```python
from build123d import *

# Parameters (mm, degrees)
F0_R          = 1.5
F0_R_2        = 4.5
F1_DEPTH      = 3
F2_W          = 12
F2_H          = 29
F3_DEPTH      = 3
F4_R          = 1.5
F5_DEPTH      = 3
F6_R          = 4
F6_R_2        = 1.5
F7_DEPTH      = 3
F9_R          = 2
F10_T4_DEPTH  = 12
F10_S5_R      = 1.5
F10_T6_DEPTH  = 8
F10_T10_DEPTH = 12
F10_S11_R     = 1.5
F10_T12_DEPTH = 8
F11_R         = 3
F12_DEPTH     = 4
F13_R         = 0.5
F14_DEPTH     = 3
F15_T1_DEPTH  = 8
F16_T1_DEPTH  = 8
F17_SIZE      = 2


# Not quite as in the source:
# - a fillet or chamfer that OpenCascade refuses, or shapes differently, is made with other operations: its cross-section is extruded or revolved along the edge and cut away or added


with BuildPart() as f1:
    # F0 (on Front) → F1 (new body)
    with BuildSketch(Plane.XZ):
        with BuildLine():
            Line((0, -5.5), (9.5, -5.5))
            ThreePointArc((9.5, -5.5), (11.6605151609, -5.0578823869), (13.4736842105, -3.8026088144))
            ThreePointArc((13.4736842105, -3.8026088144), (14, 0), (13.4736842105, 3.8026088144))
            ThreePointArc((13.4736842105, 3.8026088144), (11.6605151609, 5.0578823869), (9.5, 5.5))
            Line((9.5, 5.5), (0, 5.5))
            Line((0, 5.5), (-9.5, 5.5))
            ThreePointArc((-9.5, 5.5), (-11.6605151609, 5.0578823869), (-13.4736842105, 3.8026088144))
            ThreePointArc((-13.4736842105, 3.8026088144), (-14, 0), (-13.4736842105, -3.8026088144))
            ThreePointArc((-13.4736842105, -3.8026088144), (-11.6605151609, -5.0578823869), (-9.5, -5.5))
            Line((-9.5, -5.5), (0, -5.5))
        make_face()
        with Locations((-9.5, 0)):
            Circle(F0_R, mode=Mode.SUBTRACT)
        Circle(F0_R_2, mode=Mode.SUBTRACT)
        with Locations((9.5, 0)):
            Circle(F0_R, mode=Mode.SUBTRACT)
    extrude(amount=F1_DEPTH)

    # F2 (on face) → F3 (join)
    with BuildSketch(Plane.XZ.offset(3)):
        Rectangle(F2_W, F2_H)
    extrude(amount=-F3_DEPTH)

    # F4 (on face) → F5 (join)
    with BuildSketch(Plane(origin=(0, 0, -14.5), x_dir=(1, 0, 0), z_dir=(0, 0, -1))):
        with BuildLine():
            Line((-6, 13.5), (-6, 0))
            Line((-6, 0), (6, 0))
            Line((6, 0), (6, 13.5))
            ThreePointArc((6, 13.5), (5.1213203436, 15.6213203436), (3, 16.5))
            Line((3, 16.5), (-3, 16.5))
            ThreePointArc((-3, 16.5), (-5.1213203436, 15.6213203436), (-6, 13.5))
        make_face()
        with Locations((0, 12.5)):
            Circle(F4_R, mode=Mode.SUBTRACT)
    extrude(amount=-F5_DEPTH)

    # F6 (on face) → F7 (cut, through all)
    with BuildSketch(Plane(origin=(0, 0, 0), x_dir=(-1, 0, 0), z_dir=(0, 1, 0))):
        Circle(F6_R)
        with Locations((0, 8)):
            Circle(F6_R_2)
        with Locations((0, -8)):
            Circle(F6_R_2)
    extrude(amount=-F7_DEPTH, mode=Mode.SUBTRACT)

    # F8: F1 across plane


with BuildPart() as f1_1:
    add(f1.part)
    add(f1.part.mirror(Plane.XY))

    # F9
    f9_edges = [f1_1.edges().sort_by_distance(p)[0] for p in [
        (0, 0, 14.5),
    ]]
    fillet(f9_edges, radius=F9_R)

    # F10: chamfer of 3 on 2 edges, made by hand


with BuildPart() as f10_tool2:
    # F10_s3 → F10_t4 (new body)
    with BuildSketch(Plane.YZ.offset(-6)):
        Polygon((-3, 8.5), (-6, 11.5), (-3, 11.5), align=None)
    extrude(amount=F10_T4_DEPTH)

    # F10_s5 → F10_t6 (cut, symmetric)
    with BuildSketch(Plane.XZ.offset(4.5)):
        with Locations((0, 8)):
            Circle(F10_S5_R)
    extrude(amount=F10_T6_DEPTH, both=True, mode=Mode.SUBTRACT)


with BuildPart() as f1_2:
    add(f1_1.part)

    # F10_t1: union F10_tool2
    add(f10_tool2.part)


with BuildPart() as f10_tool8:
    # F10_s9 → F10_t10 (new body)
    with BuildSketch(Plane.YZ.offset(-6)):
        Polygon((-3, -8.5), (-6, -11.5), (-3, -11.5), align=None)
    extrude(amount=F10_T10_DEPTH)

    # F10_s11 → F10_t12 (cut, symmetric)
    with BuildSketch(Plane.XZ.offset(4.5)):
        with Locations((0, -8)):
            Circle(F10_S11_R)
    extrude(amount=F10_T12_DEPTH, both=True, mode=Mode.SUBTRACT)


with BuildPart() as f1_3:
    add(f1_2.part)

    # F10_t7: union F10_tool8
    add(f10_tool8.part)

    # F11 (on face) → F12 (cut)
    with BuildSketch(Plane.XZ.offset(3)):
        with Locations((0, 8)):
            Circle(F11_R)
        with Locations((0, -8)):
            Circle(F11_R)
    extrude(amount=F12_DEPTH, mode=Mode.SUBTRACT)

    # F13 (on face) → F14 (join)
    with BuildSketch(Plane(origin=(0, 0, -14.5), x_dir=(1, 0, 0), z_dir=(0, 0, -1))):
        with BuildLine():
            Line((-11.9, 0), (6, 0))
            Line((6, 0), (6, 8))
            Line((6, 8), (-11.9, 8))
            ThreePointArc((-11.9, 8), (-13.3849242405, 7.3849242405), (-14, 5.9))
            Line((-14, 5.9), (-14, 2.1))
            ThreePointArc((-14, 2.1), (-13.3849242405, 0.6150757595), (-11.9, 0))
        make_face()
        with Locations((-10.3164756671, 2.1835243329)):
            Circle(F13_R, mode=Mode.SUBTRACT)
        with BuildLine():
            Line((6, 8), (6, 0))
            Line((6, 0), (11.9, 0))
            ThreePointArc((11.9, 0), (13.3849242405, 0.6150757595), (14, 2.1))
            Line((14, 2.1), (14, 5.9))
            ThreePointArc((14, 5.9), (13.3849242405, 7.3849242405), (11.9, 8))
            Line((11.9, 8), (6, 8))
        make_face()
        with Locations((10.3164756671, 2.1835243329)):
            Circle(F13_R, mode=Mode.SUBTRACT)
    extrude(amount=F14_DEPTH)

    # F15: chamfer of 2 on 1 edges, made by hand

    # F15_s2 → F15_t1 (join)
    with BuildSketch(Plane.XZ):
        Polygon((-6, -12.5), (-8, -14.5), (-6, -14.5), align=None)
    extrude(amount=F15_T1_DEPTH)

    # F16: chamfer of 2 on 1 edges, made by hand

    # F16_s2 → F16_t1 (join)
    with BuildSketch(Plane.XZ):
        Polygon((8, -14.5), (6, -12.5), (6, -14.5), align=None)
    extrude(amount=F16_T1_DEPTH)

    # F17
    f17_edges = [f1_3.edges().sort_by_distance(p)[0] for p in [
        (0, -8, -14.5),
    ]]
    chamfer(f17_edges, length=F17_SIZE)


solid = f1_3.part
```
Input: part model. Units: mm. Frame: model coordinates. A direction names the side the tool comes from. Coordinates: 2 decimals unless noted, no trailing zeros. Write each loop counter-clockwise with the first axis right and the second up, starting at its lowest first coordinate (ties: lowest second). Pieces come first, ordered by that corner, then holes. Notation, with made-up numbers: (27.5, 49.25) - (33.5, 49.25) arc R24 ccw to (33.5, 68.25) - close; hole circle Ø5 at (30, -31). An arc over 180 degrees is marked (long way). Put each result on its own line as item: value. Start each with the question number.
1) Reachability of faces 4 (the face through (0, -15, -14.5)), 5 (the face through (-6, -5, 11)), 6 (the face through (6, -5, 11)) from +Z, -Z, +X, -X, +Y, -Y: full face, straight path, thin tool, end or side. Return the list, or none.
2) Contact query for flat-ended pins moving along their axis: pin 1 (12 mm diameter, centred on x = 0.5, z = 1, fed in from +Y); pin 2 (2 mm diameter, centred on x = 1, z = 9, fed in from -Y); pin 3 (3.5 mm diameter, centred on x = -8, y = -1, fed in from +Z); pin 4 (7 mm diameter, centred on y = -6, z = 8.5, fed in from +X). Output: stop coordinate, or through.
3) Ray query, L1, parallel to Z at x = 9.5, y = -1.75; L2, parallel to X at y = -12.5, z = -13.2; L3, parallel to Z at x = 0, y = -2.2. Return the intervals inside material, ascending.
4) Cut plane B-B (z = 8). Return the cut outline in (x, y), plus the area to 3 significant figures.
5) Cut plane A-A (y = -12.5). Return the cut outline in (x, z), plus the area to 3 significant figures.
6) Cut plane D-D (z = 0). Return the cut outline in (x, y).
7) Mould query, pull axis Z, two halves, no side actions, for faces 1 (the face through (-11, -4, -14.5)), 2 (the face through (14, -4, -16)), 3 (the face through (0, -9, 14.5)). Classes: pulls with the +Z half, pulls with the -Z half, needs draft (parallel to the pull), parting line crosses it, or undercut.
8) Cut plane C-C (x = -7.5). Return the cut outline in (y, z).
Resolved:
1. face 4: -Z, +X, -X, -Y
1. face 5: +Z, -X, +Y, -Y
1. face 6: +Z, +X, +Y, -Y
2. pin 1: stops at y = 0
2. pin 2: stops at y = -3
2. pin 3: stops at z = 5.5
2. pin 4: stops at x = 6
3. L1: z = -17.5 to -14.5, -5.5 to -1.5, 1.5 to 5.5
3. L2: x = -6 to -1.5, 1.5 to 6
3. L3: z = -17.5 to -9.5, -6.5 to -4, 4 to 6.5, 9.5 to 14.5
4. outline: (-6, -3) - (-1.5, -3) - (-1.5, 0) - (-6, 0) - close; (1.5, -3) - (6, -3) - (6, 0) - (1.5, 0) - close
4. area: 27.0 mm2
5. outline: (-6, -14.5) - (-1.5, -14.5) - (-1.5, -11.5) - (-6, -11.5) - close; (-6, 11.5) - (-1.5, 11.5) - (-1.5, 14.5) - (-6, 14.5) - close; (1.5, -14.5) - (6, -14.5) - (6, -11.5) - (1.5, -11.5) - close; (1.5, 11.5) - (6, 11.5) - (6, 14.5) - (1.5, 14.5) - close
5. area: 54.0 mm2
6. outline: (-14, -3) - (-11, -3) - (-11, 0) - (-14, 0) - close; (-8, -3) - (-4, -3) - (-4, 0) - (-8, 0) - close; (4, -3) - (8, -3) - (8, 0) - (4, 0) - close; (11, -3) - (14, -3) - (14, 0) - (11, 0) - close
7. face 1: undercut
7. face 2: needs draft
7. face 3: pulls with the +Z half
8. outline: (-8, -17.5) - (0, -17.5) - (0, -14) - (-8, -14) - close; (-3, -5.5) - (0, -5.5) - (0, 5.5) - (-3, 5.5) - close
